```python
from build123d import *

# Parameters (mm, degrees)
F1_DEPTH = 25.4
F3_R     = 5.08


# Not quite as in the source:
# - a feature of the source that left no trace in its solid (it failed there, or was rolled back) is left out


with BuildPart() as f1:
    # F0 (on Front) → F1 (new body)
    with BuildSketch(Plane.XZ):
        with BuildLine():
            ThreePointArc((39.115998894, 27.4320002645), (20.3391036575, 46.3696241803), (0, 29.1206747426))
            ThreePointArc((0, 29.1206747426), (-20.3391036575, 46.3696241803), (-39.115998894, 27.4320002645))
            ThreePointArc((-39.115998894, 27.4320002645), (-24.9919364346, -8.4631327613), (0, -37.8459990025))
            ThreePointArc((0, -37.8459990025), (24.9919364346, -8.4631327613), (39.115998894, 27.4320002645))
        make_face()
        with BuildLine():
            ThreePointArc((0, 29.1206747426), (0.1433513735, 26.7523380063), (0, 24.3840012699))
            ThreePointArc((0, 24.3840012699), (-0.1433513735, 26.7523380063), (0, 29.1206747426))
        make_face(mode=Mode.SUBTRACT)
        with BuildLine():
            ThreePointArc((0, 29.1206747426), (-0.1433513735, 26.7523380063), (0, 24.3840012699))
            ThreePointArc((0, 24.3840012699), (0.1433513735, 26.7523380063), (0, 29.1206747426))
        make_face()
    extrude(amount=F1_DEPTH)

    # F3
    f3_edges = [f1.edges().sort_by_distance(p)[0] for p in [
        (20.339104, 0, 46.369624),
        (20.339104, -25.4, 46.369624),
        (0, -12.7, 29.120675),
        (-39.115999, -12.7, 27.432),
        (-20.339104, 0, 46.369624),
        (-20.339104, -25.4, 46.369624),
        (39.115999, -12.7, 27.432),
        (-24.991936, 0, -8.463133),
        (-24.991936, -25.4, -8.463133),
        (24.991936, 0, -8.463133),
        (24.991936, -25.4, -8.463133),
    ]]
    fillet(f3_edges, radius=F3_R)


solid = f1.part
```
Verification items for the finished model (mm, model axes). Coordinates: 2 decimals unless noted, no trailing zeros. Loops run counter-clockwise (first coordinate to the right, second up) from the corner with the lowest first, then second, coordinate; pieces in that order, holes last. Notation, with made-up numbers: (46, 21) - (95, 21) arc R26 cw to (95, 54) - close; hole circle Ø4 at (26.25, 54.25). An arc over 180 degrees is marked (long way). Put each result on its own line as item: value.
Item 1: Gauge pin test, flat ends, axial feed: pin 1 Ø2 at (x, y) = (27.5, -8.5) entering from -Z; pin 2 Ø10 at (y, z) = (-12, -9) entering from -X; pin 3 Ø6 at (y, z) = (-11.5, 1) entering from -X; pin 4 Ø1 at (x, z) = (-26, 32) entering from +Y. Record the tip position at first contact, or that the pin passes through.
Conclusion:
pin 1: stops at z = -5.87
pin 2: stops at x = -27.54
pin 3: stops at x = -31.48
pin 4: stops at y = 0
Item 2: Section check A-A (y = -2). Enter the section's corners in (x, z).
Conclusion:
outline: (-38.04, 28.14) arc R4.04 ccw to (-37.95, 26.98) arc R116.4 ccw to (0, -36.48) arc R116.4 ccw to (37.95, 26.98) arc R4.04 ccw to (38.04, 28.14) arc R18.6 ccw to (4.83, 38.19) arc R6.12 cw to (-4.83, 38.19) arc R18.6 ccw to start
Item 3: Draft check along X on faces 1 (the face through (-24.86, -12.59, 45.64)), 2 (the face through (24.534, -12.593, -9.221)), 3 (the face through (0, -25.4, 14)). Enter one of: pulls with the +X half, pulls with the -X half, needs draft (parallel to the pull), parting line crosses it, or undercut.
Conclusion:
face 1: undercut
face 2: pulls with the +X half
face 3: needs draft
Item 4: Scan lines: line 1 along X through (y, z) = (-8.5, 41.5); line 2 along X through (y, z) = (-4, 41); line 3 along Z through (x, y) = (-11, -15.25). Record each from-to range of solid material in increasing order.
Conclusion:
line 1: x = -32.46 to -6.53, 6.53 to 32.46
line 2: x = -32.83 to -6.15, 6.15 to 32.83
line 3: z = -27.26 to 44.46
